Can you work these out from the model? Positions are in its coordinate system, mm. Face numbers are marked on the shaded views. A direction names the side the tool comes from. Coordinates: 2 decimals unless noted, no trailing zeros. Write each loop counter-clockwise with the first axis right and the second up, starting at its lowest first coordinate (ties: lowest second). Pieces come first, ordered by that corner, then holes. Notation, with made-up numbers: (63, 11.25) -> (74, 11.25) arc R20 cw to (74, 42.25) -> close; hole circle Ø2 at (68, -18). An arc over 180 degrees is marked (long way). Use one line per item in the form item = value.
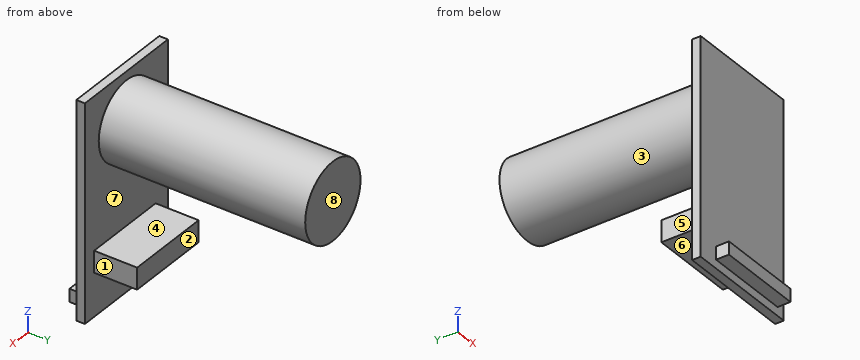
Autodesk Fusion 360 part; units mm, degrees
sketch "Skizze1" plane through (0, 0, 0) normal (0, 1, 0) x (1, 0, 0)
  line L0 (0, 0) -> (27, 0)
  line L1 (27, 0) -> (27, -50)
  line L2 (27, -50) -> (0, -50)
  line L3 (0, -50) -> (0, 0)
  line L4 (13.5, -50) -> (13.5, -39)
  circle A0 centre (13.5, -39) radius 9
  dimension "d1" = 50
  dimension "d2" = 27
  dimension "d3" = 11
  dimension "d4" = 18
extrude "Extrusion1" add sketch "Skizze1" along normal blind 50 contours A0 makes body 1
extrude "Extrusion2" add sketch "Skizze1" along normal blind 2 bodies 1
sketch "Skizze2" plane through (0, 2, 0) normal (0, 1, 0) x (-1, 0, 0)
  circle A0 centre (-13.5, 39) radius 9
  line L0 (0, 50) -> (-27, 50)
  line L1 (-27, 50) -> (-27, 0)
  line L2 (-27, 0) -> (0, 0)
  line L3 (0, 0) -> (0, 50)
  line L4 (0, 0) -> (-4, 0)
  line L5 (-4, 0) -> (-4, 10)
  line L6 (-4, 10) -> (0, 10)
  line L7 (0, 10) -> (0, 0)
  line L8 (-4, 10) -> (-24, 10)
  line L9 (-24, 10) -> (-24, 15)
  line L10 (-24, 15) -> (-4, 15)
  line L11 (-4, 15) -> (-4, 10)
  dimension "d9" = 10
  dimension "d10" = 4
  dimension "d11" = 20
  dimension "d12" = 5
extrude "Extrusion3" add sketch "Skizze2" along normal blind 10 contours L8 L9 L10 L11 bodies 1
sketch "Skizze3" plane through (0, 2, 0) normal (0, 1, 0) x (-1, 0, 0)
  line L0 (-4, 15) -> (-4, 10)
  line L1 (-4, 10) -> (-24, 10)
  line L2 (-24, 10) -> (-24, 15)
  line L3 (-24, 15) -> (-4, 15)
  circle A0 centre (-13.5, 39) radius 9
  line L4 (0, 50) -> (-27, 50)
  line L5 (-27, 50) -> (-27, 0)
  line L6 (-27, 0) -> (0, 0)
  line L7 (0, 0) -> (0, 50)
  line L8 (-5, 5) -> (-25, 5)
  line L9 (-25, 5) -> (-25, 2)
  line L10 (-25, 2) -> (-5, 2)
  line L11 (-5, 2) -> (-5, 5)
  dimension "d15" = 20
  dimension "d16" = 3
extrude "Extrusion4" add sketch "Skizze3" against normal blind 5 contours L8 L9 L10 L11 bodies 1
copy_body "Körper->Berechn1" bodies 1 removing the originals makes body 2 in component "nixie_modul"
component "nixie_modul" placed x (1, 0, 0) y (0, 1, 0) z (0, 0, 1) at (0, 0, 0)
Q1. If I drill on line 1 (Y direction, x = 3.75, z = 48); line 2 (X direction, y = 8, z = 11); line 3 (Y direction, x = 19, z = 36), over which ranges is the centre line in solid material (lowest first)? Write a range as from..to.
Return value:
line_1 = 0..2
line_2 = 4..24
line_3 = 0..50
Q2. Suppose I cut it at A-A (x = 13.5). Write out the boundary of the cut face in (y, z).
Return value:
outline = (-3, 2) -> (0, 2) -> (0, 0) -> (2, 0) -> (2, 10) -> (12, 10) -> (12, 15) -> (2, 15) -> (2, 30) -> (50, 30) -> (50, 48) -> (2, 48) -> (2, 50) -> (0, 50) -> (0, 5) -> (-3, 5) -> close
Q3. Will these pins go through, and if not, where does the flat tip stop? pin 1 (4 mm diameter, centred on y = 7, z = 12, fed in from +X); pin 2 (11 mm diameter, centred on x = 19, y = 5.5, fed in from -Z); pin 3 (2 mm diameter, centred on x = 3, z = 34, fed in from -Y); pin 4 (2.5 mm diameter, centred on x = 15, y = -1.5, fed in from +Z).
Return value:
pin_1 = 24
pin_2 = 0
pin_3 = 0
pin_4 = 5
Q4. For the marked faces 1, 2, 3, 4 and 5, which set-ups out of +Z, -Z, +X, -X, +Y, -Y let a thin tool reach every point of the face, with its end or its side?
Return value:
face_1 = +Z, -Z, +X, +Y
face_2 = -Z, +X, -X, +Y
face_3 = +Y
face_4 = +X, -X, +Y
face_5 = +Z, -Z, -X, +Y
Q5. Suppose I cut it at D-D (z = 39). Write out the boundary of the cut face in (x, y).
Return value:
outline = (0, 0) -> (27, 0) -> (27, 2) -> (22.5, 2) -> (22.5, 50) -> (4.5, 50) -> (4.5, 2) -> (0, 2) -> close
Q6. Suppose I cut it at C-C (y = 38). Write out the boundary of the cut face in (x, z).
Return value:
outline = circle Ø18 at (13.5, 39)
Q7. Thinking about a two-plate mould opening in Z: for the marked faces 6, 7 and 8, which applies, released by +Z, released by -Z, zero draft, split by the parting line, or undercut?
Return value:
face_6 = released by -Z
face_7 = undercut
face_8 = zero draft
Q8. Suppose I cut it at B-B (z = 12). Write out the boundary of the cut face in (x, y).
Return value:
outline = (0, 0) -> (27, 0) -> (27, 2) -> (24, 2) -> (24, 12) -> (4, 12) -> (4, 2) -> (0, 2) -> close
